Read the model definition and answer for the solid it produces. Units are mm, in the model's axes. A direction names the side the tool comes from. Give positions to 0.01 mm unless a question says otherwise; leave off trailing zeros. Loops run counter-clockwise (first coordinate to the right, second up) from the corner with the lowest first, then second, coordinate; pieces in that order, holes last. Notation, with made-up numbers: (76, -19.75) - (98, -19.75) arc R19 cw to (98, -2.75) - close; hole circle Ø7 at (6.25, 13.25). An arc over 180 degrees is marked (long way). Write each question's results on one line, items separated by ' | '. Start each with the question number.
Q1. For faces 1 (the flat face through (93, 12.5, -75)), 2 (the flat face through (-93, 12.5, -75)), 3 (the flat face through (-86.5, 9, -75)), determine the directions among +Z, -Z, +X, -X, +Y, -Y from which every point of the face is accessible in a straight line to the end or side of a thin tool.
Q2. Find the intervals of material crossed by line 1 (X direction, y = 4.5, z = -64); line 2 (X direction, y = 11.75, z = -78.5); line 3 (X direction, y = 16, z = -83), in increasing order. Write a range as from..to.
Q3. Given pin 1 (1.8 mm diameter, centred on x = -88, z = -72.5, fed in from +Y); pin 2 (0.7 mm diameter, centred on x = 88, z = -80, fed in from +Y), each flat-ended and moving along its own axis, determine where each tip first touches the part or whether it passes through.
Q4. The part is cut by section A-A, the plane z = -77.5. Write down the section's boundary in (x, y).
```python
from build123d import *

# Parameters (mm, degrees)
BOSS_EXTRUDE1_DEPTH      = 19.25
BOSS_EXTRUDE1_DEPTH_BACK = 5
SKETCH1_W                = 173
SKETCH1_H                = 25
SKETCH2_W                = 15
SKETCH2_H                = 25
BOSS_EXTRUDE2_DEPTH      = 5
SKETCH3_W                = 12.75
SKETCH3_H                = 25
BOSS_EXTRUDE3_DEPTH      = 12.5
FILLET1_R                = 5


with BuildPart() as part:
    # Sketch1 → Boss-Extrude1 (new, two sides: drawn at the far end of the back side and taken through both)
    with BuildSketch(Plane(origin=(0, 0, 0), x_dir=(1, 0, 0), z_dir=(0, 1, 0)).offset(-BOSS_EXTRUDE1_DEPTH_BACK)):
        with Locations((0, 75)):
            Rectangle(SKETCH1_W, SKETCH1_H)
    extrude(amount=BOSS_EXTRUDE1_DEPTH + BOSS_EXTRUDE1_DEPTH_BACK)

    # Sketch2 → Boss-Extrude2 (add)
    with BuildSketch(Plane(origin=(0, -5, 0), x_dir=(1, 0, 0), z_dir=(0, 1, 0))):
        with Locations((-94, 75)):
            Rectangle(SKETCH2_W, SKETCH2_H)
        with Locations((94, 75)):
            Rectangle(SKETCH2_W, SKETCH2_H)
    extrude(amount=BOSS_EXTRUDE2_DEPTH)

    # Sketch3 → Boss-Extrude3 (add)
    with BuildSketch(Plane(origin=(0, 0, 0), x_dir=(1, 0, 0), z_dir=(0, 1, 0))):
        with Locations((-95.125, 75)):
            Rectangle(SKETCH3_W, SKETCH3_H)
        with Locations((95.125, 75)):
            Rectangle(SKETCH3_W, SKETCH3_H)
    extrude(amount=BOSS_EXTRUDE3_DEPTH)

    # Fillet1
    fillet1_edges = [part.edges().sort_by_distance(p)[0] for p in [
        (-101.5, -5, -75),
        (101.5, -5, -75),
        (-101.5, 12.5, -75),
        (101.5, 12.5, -75),
    ]]
    fillet(fillet1_edges, radius=FILLET1_R)


solid = part.part
```
Check sheet entries:
1) face 1: +Z, -Z, +X, +Y | face 2: +Z, -Z, -X, +Y | face 3: +Z, -Z, +Y
2) line 1: x = -101.5..-88.75, -86.5..86.5, 88.75..101.5 | line 2: x = -99.13..-88.75, -86.5..86.5, 88.75..99.13 | line 3: x = -86.5..86.5
3) pin 1: stops at y = 12.5 | pin 2: stops at y = 0
4) outline: (-101.5, 0) arc R5 ccw to (-96.5, -5) - (96.5, -5) arc R5 ccw to (101.5, 0) - (101.5, 7.5) arc R5 ccw to (96.5, 12.5) - (88.75, 12.5) - (88.75, 0) - (86.5, 0) - (86.5, 19.25) - (-86.5, 19.25) - (-86.5, 0) - (-88.75, 0) - (-88.75, 12.5) - (-96.5, 12.5) arc R5 ccw to (-101.5, 7.5) - close
